Read the model definition and answer for the solid it produces. Units are mm, in the model's axes. Face numbers are marked on the shaded views. A direction names the side the tool comes from. Give positions to 0.01 mm unless a question says otherwise; leave off trailing zeros. Order: outer loops, then holes, each group sorted by start corner. A loop starts at its lowest first (then second) coordinate and runs counter-clockwise, first axis right, second up. Notation, with made-up numbers: (4.25, 49.25) - (38.25, 49.25) arc R31 ccw to (38.25, 73.25) - close; hole circle Ø11 at (7, 73.25). An arc over 180 degrees is marked (long way). Write each question's results on one line, items separated by ' | '.
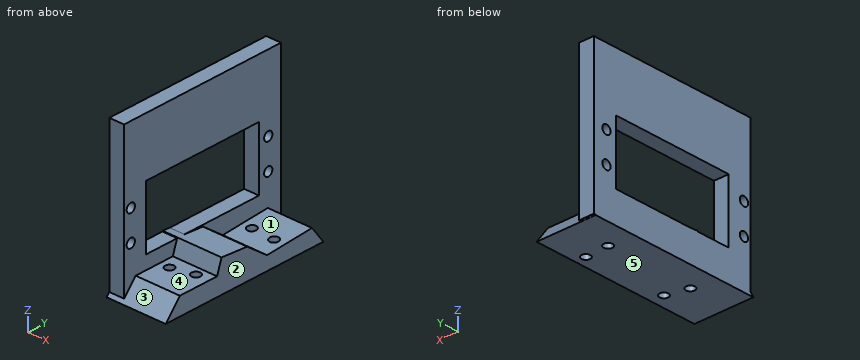
from build123d import *

# Parameters (mm, degrees)
SKETCH010_R   = 1.5
PAD006_DEPTH  = 100
PAD005_DEPTH  = 20
SKETCH008_W   = 57.061168
SKETCH008_H   = 50.408328
SKETCH008_R   = 1.5
SKETCH008_W_2 = 41.061168
SKETCH008_H_2 = 20.879282
PAD004_DEPTH  = 5


with BuildPart() as screwcutouts:
    # Sketch010 → Pad006 (new body)
    with BuildSketch(Plane.XY):
        with Locations((40.429066, 8.263429)):
            Circle(SKETCH010_R)
        with Locations((48.370731, 7.858237)):
            Circle(SKETCH010_R)
        with Locations((40.348022, -21.55835)):
            Circle(SKETCH010_R)
        with Locations((47.560356, -19.694489)):
            Circle(SKETCH010_R)
    extrude(amount=-PAD006_DEPTH)


with BuildPart() as mountsupportpad:
    # Sketch009 → Pad005 (new body)
    with BuildSketch(Plane.YZ.offset(32)):
        Polygon((-35.508293, -20.850826), (-30.321894, -14.935085), (-16.788631, -14.935085), (-15.16788, -10.234911), (-5.848567, -10.964246), (1.363771, -16.312723), (17.733341, -15.259238), (21.866251, -20.850826), align=None)
    extrude(amount=PAD005_DEPTH)


with BuildPart() as cut003:
    # Sketch008 → Pad004 (new body)
    with BuildSketch(Plane.YZ.offset(32)):
        with Locations((-6.005477, 4.48483)):
            Rectangle(SKETCH008_W, SKETCH008_H)
        with Locations((-32.087313, 5.013472)):
            Circle(SKETCH008_R, mode=Mode.SUBTRACT)
        with Locations((-32.087313, -4.986528)):
            Circle(SKETCH008_R, mode=Mode.SUBTRACT)
        with Locations((17.912687, 5.013472)):
            Circle(SKETCH008_R, mode=Mode.SUBTRACT)
        with Locations((17.912687, -4.986528)):
            Circle(SKETCH008_R, mode=Mode.SUBTRACT)
        with Locations((-6.005477, 0)):
            Rectangle(SKETCH008_W_2, SKETCH008_H_2, mode=Mode.SUBTRACT)
    extrude(amount=PAD004_DEPTH)

    # Fusion003: union MountSupportPad
    add(mountsupportpad.part)

    # Cut003: cut ScrewCutouts
    add(screwcutouts.part, mode=Mode.SUBTRACT)


solid = cut003.part
(1) Each of these flat-tipped pins is pushed along its axis until it touches: pin 1 (10 mm diameter, centred on y = 13.5, z = -4.5, fed in from +X); pin 2 (2.5 mm diameter, centred on x = 48.37, y = 7.86, fed in from +Z); pin 3 (4 mm diameter, centred on x = 45.5, y = -21, fed in from +Z); pin 4 (1.5 mm diameter, centred on x = 34, z = 0.5, fed in from -Y). Where does it stop, or does it pass through?
Conclusion:
pin 1: x = 37 | pin 2: through | pin 3: z = -14.94 | pin 4: y = -34.54
(2) Consider probe 1 along Y at (x, z) = (36.5, -9); probe 2 along Y at (x, z) = (40.25, -17); probe 3 along X at (y, z) = (-15, 26.5). Determine where each line is inside the solid, lowest interval first. Write a range as [from, to].
Conclusion:
probe 1: [-34.54, -26.54], [14.53, 22.53] | probe 2: [-32.13, -23.06], [-20.06, 6.77], [9.75, 19.02] | probe 3: [32, 37]
(3) Section D-D (y = -28) is taken. Give the vertices of the cut face in (x, z).
Conclusion:
outline: (32, -20.85) - (52, -20.85) - (52, -14.94) - (37, -14.94) - (37, 29.69) - (32, 29.69) - close
(4) Section B-B (y = -14) is taken. Give the vertices of the cut face in (x, z).
Conclusion:
outline: (32, -20.85) - (52, -20.85) - (52, -10.33) - (32, -10.33) - close; (32, 10.44) - (37, 10.44) - (37, 29.69) - (32, 29.69) - close
(5) The mould has two halves that part along Y. Classify the marked faces 1, 2 and 3: pulls with the +Y half, pulls with the -Y half, needs draft (parallel to the pull), parting line crosses it, or undercut.
Conclusion:
face 1: undercut | face 2: needs draft | face 3: pulls with the -Y half
(6) Section A-A (z = -7.5) is taken. Give the vertices of the cut face in (x, y), plus the area to 3 significant figures.
Conclusion:
outline: (32, -34.54) - (37, -34.54) - (37, -26.54) - (32, -26.54) - close; (32, 14.53) - (37, 14.53) - (37, 22.53) - (32, 22.53) - close | area: 80.0 mm^2
(7) For the marked faces 4 and 5, determine the directions among +Z, -Z, +X, -X, +Y, -Y from which every point of the face is accessible in a straight line to the end or side of a thin tool.
Conclusion:
face 4: +Z, +X, -Y | face 5: -Z, +X, -X, +Y, -Y
(8) Section C-C (x = 40) is taken. Give the vertices of the cut face in (y, z).
Conclusion:
outline: (-35.51, -20.85) - (-23.02, -20.85) - (-23.02, -14.94) - (-30.32, -14.94) - close; (-20.1, -20.85) - (6.83, -20.85) - (6.83, -15.96) - (1.36, -16.31) - (-5.85, -10.96) - (-15.17, -10.23) - (-16.79, -14.94) - (-20.1, -14.94) - close; (9.7, -20.85) - (21.87, -20.85) - (17.73, -15.26) - (9.7, -15.78) - close
